```python
from build123d import *

# Parameters (mm, degrees)
F0_R     = 1.45
F1_DEPTH = 2


with BuildPart() as f1:
    # F0 (on Top) → F1 (new body)
    with BuildSketch(Plane.XY):
        with BuildLine():
            Line((16.0432131672, 48.2310554204), (13.0458830723, 48.2310554204))
            ThreePointArc((13.0458830723, 48.2310554204), (10.9245627287, 47.352375764), (10.0458830723, 45.2310554204))
            Line((10.0458830723, 45.2310554204), (10.0458830723, 23.7476840101))
            add(Edge.make_bspline(
                [(10.0458830723, 23.7476840101), (10.7115456302, 22.4846217094), (11.005823731, 20.7161298766), (10.3430984406, 19.7198280209), (9.2372713755, 19.6688592385)],
                knots=[0, 0, 0, 0, 0.5644517657, 1, 1, 1, 1], degree=3))
            add(Edge.make_bspline(
                [(9.3841085265, 20.9630623411), (9.4691643546, 20.7871442379), (8.4748883735, 20.4145718213), (8.6683240442, 19.7080140495), (9.2372713755, 19.6688592385)],
                knots=[0, 0, 0, 0, 0.5139461709, 1, 1, 1, 1], degree=3))
            Line((9.3841085265, 20.9630623411), (8.2844858954, 20.9630623411))
            Line((8.2844858954, 20.9630623411), (7.8372713755, 20.9630623411))
            Line((7.8372713755, 20.9630623411), (7.8372713755, 18.9225599587))
            Line((7.8372713755, 18.9225599587), (26.3372713755, 18.9225599587))
            Line((26.3372713755, 18.9225599587), (26.3372713755, 44.1340877949))
            add(Edge.make_bspline(
                [(16.0432131672, 48.2310554204), (17.9878656476, 47.6235912963), (21.4636227702, 44.1599026946), (24.841907136, 44.140700061), (26.3372713755, 44.1340877949)],
                knots=[0.341159936, 0.341159936, 0.341159936, 0.341159936, 0.6993169326, 1, 1, 1, 1], degree=3))
        make_face()
        with BuildLine():
            add(Edge.make_bspline(
                [(23.8372713755, 38.432449385), (22.5156090399, 38.7503102684), (22.055353444, 39.0385909711), (19.4297470837, 40.8717350173), (17.8784877062, 41.6118882482)],
                knots=[0.0042165568, 0.0042165568, 0.0042165568, 0.0042165568, 0.4134444878, 1, 1, 1, 1], degree=3))
            Line((23.8372713755, 38.432449385), (23.8372713755, 23.1634433148))
            Line((23.8372713755, 23.1634433148), (23.8372713755, 21.4225599587))
            Line((23.8372713755, 21.4225599587), (22.228775843, 21.4225599587))
            Line((22.228775843, 21.4225599587), (20.3372713755, 21.4225599587))
            ThreePointArc((20.3372713755, 21.4225599587), (18.5695044225, 22.1547930057), (17.8372713755, 23.9225599587))
            Line((17.8372713755, 23.9225599587), (17.8372713755, 38.9225599587))
            Line((17.8372713755, 38.9225599587), (17.8691951823, 41.617109993))
            Line((17.8691951823, 41.617109993), (17.8784877062, 41.6118882482))
        make_face(mode=Mode.SUBTRACT)
        with Locations((14.9654557983, 38.6260170906)):
            Circle(F0_R, mode=Mode.SUBTRACT)
        with BuildLine():
            add(Edge.make_bspline(
                [(36.6313295837, 48.2310554204), (34.6866771033, 47.6235912963), (31.2109199807, 44.1599026946), (27.8326356149, 44.140700061), (26.3372713755, 44.1340877949)],
                knots=[0.341159936, 0.341159936, 0.341159936, 0.341159936, 0.6993169326, 1, 1, 1, 1], degree=3))
            Line((26.3372713755, 44.1340877949), (26.3372713755, 18.9225599587))
            Line((26.3372713755, 18.9225599587), (44.8372713755, 18.9225599587))
            Line((44.8372713755, 18.9225599587), (44.8372713755, 20.9630623411))
            Line((44.8372713755, 20.9630623411), (44.3900568555, 20.9630623411))
            Line((44.3900568555, 20.9630623411), (43.2904342244, 20.9630623411))
            add(Edge.make_bspline(
                [(43.2904342244, 20.9630623411), (43.2053783963, 20.7871442379), (44.1996543774, 20.4145718213), (44.0062187067, 19.7080140495), (43.4372713755, 19.6688592385)],
                knots=[0, 0, 0, 0, 0.5139461709, 1, 1, 1, 1], degree=3))
            add(Edge.make_bspline(
                [(42.6286596786, 23.7476840101), (41.9629971207, 22.4846217094), (41.6687190199, 20.7161298766), (42.3314443103, 19.7198280209), (43.4372713755, 19.6688592385)],
                knots=[0, 0, 0, 0, 0.5644517657, 1, 1, 1, 1], degree=3))
            Line((42.6286596786, 23.7476840101), (42.6286596786, 45.2310554204))
            ThreePointArc((42.6286596786, 45.2310554204), (41.7499800222, 47.352375764), (39.6286596786, 48.2310554204))
            Line((39.6286596786, 48.2310554204), (36.6313295837, 48.2310554204))
        make_face()
        with BuildLine():
            add(Edge.make_bspline(
                [(28.8372713755, 38.432449385), (30.158933711, 38.7503102684), (30.619189307, 39.0385909711), (33.2447956672, 40.8717350173), (34.7960550447, 41.6118882482)],
                knots=[0.0042165568, 0.0042165568, 0.0042165568, 0.0042165568, 0.4134444878, 1, 1, 1, 1], degree=3))
            Line((34.7960550447, 41.6118882482), (34.8053475686, 41.617109993))
            Line((34.8053475686, 41.617109993), (34.8372713755, 38.9225599587))
            Line((34.8372713755, 38.9225599587), (34.8372713755, 23.9225599587))
            ThreePointArc((34.8372713755, 23.9225599587), (34.1050383284, 22.1547930057), (32.3372713755, 21.4225599587))
            Line((32.3372713755, 21.4225599587), (30.4457669079, 21.4225599587))
            Line((30.4457669079, 21.4225599587), (28.8372713755, 21.4225599587))
            Line((28.8372713755, 21.4225599587), (28.8372713755, 23.1634433148))
            Line((28.8372713755, 23.1634433148), (28.8372713755, 38.432449385))
        make_face(mode=Mode.SUBTRACT)
        with Locations((37.7090869526, 38.6260170906)):
            Circle(F0_R, mode=Mode.SUBTRACT)
        with BuildLine():
            Line((44.8372713755, 18.9225599587), (26.3372713755, 18.9225599587))
            Line((26.3372713755, 18.9225599587), (26.3372713755, -6.2889678775))
            add(Edge.make_bspline(
                [(36.6313295837, -10.3859355031), (34.6866771033, -9.7784713789), (31.2109199807, -6.3147827772), (27.8326356149, -6.2955801437), (26.3372713755, -6.2889678775)],
                knots=[0.341159936, 0.341159936, 0.341159936, 0.341159936, 0.6993169326, 1, 1, 1, 1], degree=3))
            Line((36.6313295837, -10.3859355031), (39.6286596786, -10.3859355031))
            ThreePointArc((39.6286596786, -10.3859355031), (41.7499800222, -9.5072558467), (42.6286596786, -7.3859355031))
            Line((42.6286596786, -7.3859355031), (42.6286596786, 14.0974359072))
            add(Edge.make_bspline(
                [(42.6286596786, 14.0974359072), (41.9629971207, 15.3604982079), (41.6687190199, 17.1289900407), (42.3314443103, 18.1252918964), (43.4372713755, 18.1762606788)],
                knots=[0, 0, 0, 0, 0.5644517657, 1, 1, 1, 1], degree=3))
            add(Edge.make_bspline(
                [(43.2904342244, 16.8820575762), (43.2053783963, 17.0579756794), (44.1996543774, 17.430548096), (44.0062187067, 18.1371058678), (43.4372713755, 18.1762606788)],
                knots=[0, 0, 0, 0, 0.5139461709, 1, 1, 1, 1], degree=3))
            Line((43.2904342244, 16.8820575762), (44.3900568555, 16.8820575762))
            Line((44.3900568555, 16.8820575762), (44.8372713755, 16.8820575762))
            Line((44.8372713755, 16.8820575762), (44.8372713755, 18.9225599587))
        make_face()
        with Locations((37.7090869526, -0.7808971733)):
            Circle(F0_R, mode=Mode.SUBTRACT)
        with BuildLine():
            Line((34.8053475686, -3.7719900757), (34.7960550447, -3.7667683309))
            add(Edge.make_bspline(
                [(28.8372713755, -0.5873294677), (30.158933711, -0.9051903511), (30.619189307, -1.1934710537), (33.2447956672, -3.0266151), (34.7960550447, -3.7667683309)],
                knots=[0.0042165568, 0.0042165568, 0.0042165568, 0.0042165568, 0.4134444878, 1, 1, 1, 1], degree=3))
            Line((28.8372713755, -0.5873294677), (28.8372713755, 14.6816766025))
            Line((28.8372713755, 14.6816766025), (28.8372713755, 16.4225599587))
            Line((28.8372713755, 16.4225599587), (30.4457669079, 16.4225599587))
            Line((30.4457669079, 16.4225599587), (32.3372713755, 16.4225599587))
            ThreePointArc((32.3372713755, 16.4225599587), (34.1050383284, 15.6903269116), (34.8372713755, 13.9225599587))
            Line((34.8372713755, 13.9225599587), (34.8372713755, -1.0774400413))
            Line((34.8372713755, -1.0774400413), (34.8053475686, -3.7719900757))
        make_face(mode=Mode.SUBTRACT)
        with BuildLine():
            Line((26.3372713755, -6.2889678775), (26.3372713755, 18.9225599587))
            Line((26.3372713755, 18.9225599587), (7.8372713755, 18.9225599587))
            Line((7.8372713755, 18.9225599587), (7.8372713755, 16.8820575762))
            Line((7.8372713755, 16.8820575762), (8.2844858954, 16.8820575762))
            Line((8.2844858954, 16.8820575762), (9.3841085265, 16.8820575762))
            add(Edge.make_bspline(
                [(9.3841085265, 16.8820575762), (9.4691643546, 17.0579756794), (8.4748883735, 17.430548096), (8.6683240442, 18.1371058678), (9.2372713755, 18.1762606788)],
                knots=[0, 0, 0, 0, 0.5139461709, 1, 1, 1, 1], degree=3))
            add(Edge.make_bspline(
                [(10.0458830723, 14.0974359072), (10.7115456302, 15.3604982079), (11.005823731, 17.1289900407), (10.3430984406, 18.1252918964), (9.2372713755, 18.1762606788)],
                knots=[0, 0, 0, 0, 0.5644517657, 1, 1, 1, 1], degree=3))
            Line((10.0458830723, 14.0974359072), (10.0458830723, -7.3859355031))
            ThreePointArc((10.0458830723, -7.3859355031), (10.9245627287, -9.5072558467), (13.0458830723, -10.3859355031))
            Line((13.0458830723, -10.3859355031), (16.0432131672, -10.3859355031))
            add(Edge.make_bspline(
                [(16.0432131672, -10.3859355031), (17.9878656476, -9.7784713789), (21.4636227702, -6.3147827772), (24.841907136, -6.2955801437), (26.3372713755, -6.2889678775)],
                knots=[0.341159936, 0.341159936, 0.341159936, 0.341159936, 0.6993169326, 1, 1, 1, 1], degree=3))
        make_face()
        with Locations((14.9654557983, -0.7808971733)):
            Circle(F0_R, mode=Mode.SUBTRACT)
        with BuildLine():
            add(Edge.make_bspline(
                [(23.8372713755, -0.5873294677), (22.5156090399, -0.9051903511), (22.055353444, -1.1934710537), (19.4297470837, -3.0266151), (17.8784877062, -3.7667683309)],
                knots=[0.0042165568, 0.0042165568, 0.0042165568, 0.0042165568, 0.4134444878, 1, 1, 1, 1], degree=3))
            Line((17.8784877062, -3.7667683309), (17.8691951823, -3.7719900757))
            Line((17.8691951823, -3.7719900757), (17.8372713755, -1.0774400413))
            Line((17.8372713755, -1.0774400413), (17.8372713755, 13.9225599587))
            ThreePointArc((17.8372713755, 13.9225599587), (18.5695044225, 15.6903269116), (20.3372713755, 16.4225599587))
            Line((20.3372713755, 16.4225599587), (22.228775843, 16.4225599587))
            Line((22.228775843, 16.4225599587), (23.8372713755, 16.4225599587))
            Line((23.8372713755, 16.4225599587), (23.8372713755, 14.6816766025))
            Line((23.8372713755, 14.6816766025), (23.8372713755, -0.5873294677))
        make_face(mode=Mode.SUBTRACT)
    extrude(amount=F1_DEPTH)


solid = f1.part
```
Check sheet for the modelled part. Datum: model origin and axes. Units: mm. A direction names the side the tool comes from. Give positions to 0.01 mm unless a question says otherwise; leave off trailing zeros. Write each loop counter-clockwise with the first axis right and the second up, starting at its lowest first coordinate (ties: lowest second). Pieces come first, ordered by that corner, then holes.
Item 1: Cross-section at C-C (x = 34). Count the separate pieces of the cut face and the enclosed holes in it, and give its area (3 significant figures).
Item 2: Cross-section at B-B (y = 43). Enter the section's corners in (x, z), and give its area (3 significant figures).
Item 3: Access from +Z, -Z, +X, -X, +Y, -Y to the whole of each face (thin tool, end or side, straight path). Record for faces 4 (the face through (34.837, 7, 1)), 5 (the face through (9, 16.882, 1)), 6 (the face through (9, 20.963, 1)), 7 (the face through (44, 16.882, 1)).
Item 4: Gauge pin test, flat ends, axial feed: pin 1 (1 mm diameter, centred on y = 7.5, z = 0.5, fed in from -X); pin 2 (1 mm diameter, centred on x = 31, z = 0.5, fed in from +Y); pin 3 (0.6 mm diameter, centred on y = 10.5, z = 0.5, fed in from +X); pin 4 (4.5 mm diameter, centred on x = 37.71, y = -0.78, fed in from +Z). Record the tip position at first contact, or that the pin passes through.
Item 5: Cross-section at A-A (y = 7). Enter the section's corners in (x, z), and give its area (3 significant figures).
Item 6: Scan lines: L1, parallel to X at y = 37, z = 1.5; L2, parallel to Y at x = 37, z = 0.7; L3, parallel to Y at x = 32, z = 0.6. Record each from-to range of solid material in increasing order.
Item 7: Draft check along Y on faces 1 (the face through (15, 48.231, 1)), 2 (the face through (44.837, 19, 1)), 3 (the face through (34.085, 15.71, 0.986)). Enter one of: released by +Y, released by -Y, zero draft, split by the parting line, or undercut.
Report:
1. separate pieces: 3
1. enclosed holes: 0
1. area: 35.0 mm2
2. outline: (10.05, 0) - (42.63, 0) - (42.63, 2) - (10.05, 2) - close
2. area: 65.2 mm2
3. face 4: +Z, -Z
3. face 5: +Z, -Z, -X, -Y
3. face 6: +Z, -Z, -X, +Y
3. face 7: +Z, -Z, +X, -Y
4. pin 1: stops at x = 10.05
4. pin 2: stops at y = 45.17
4. pin 3: stops at x = 42.63
4. pin 4: stops at z = 2
5. outline: (10.05, 0) - (17.84, 0) - (17.84, 2) - (10.05, 2) - close; (23.84, 0) - (28.84, 0) - (28.84, 2) - (23.84, 2) - close; (34.84, 0) - (42.63, 0) - (42.63, 2) - (34.84, 2) - close
5. area: 41.2 mm2
6. L1: x = 10.05 to 17.84, 23.84 to 28.84, 34.84 to 42.63
6. L2: y = -10.39 to -2.05, 0.48 to 37.36, 39.89 to 48.23
6. L3: y = -7.62 to -2.15, 16.42 to 21.42, 39.99 to 45.46
7. face 1: released by +Y
7. face 2: zero draft
7. face 3: undercut
